Geometry check sheet. Reference: the model listing, model coordinates, mm. A direction names the side the tool comes from. Round coordinates to 2 decimals unless told otherwise and drop trailing zeros. Order: outer loops, then holes, each group sorted by start corner. A loop starts at its lowest first (then second) coordinate and runs counter-clockwise, first axis right, second up. Notation, with made-up numbers: (28.25, 84) - (47.25, 84) arc R23 cw to (47.25, 96) - close; hole circle Ø5 at (-8.5, 74.25). An arc over 180 degrees is marked (long way). Write each question's results on one line, items separated by ' | '.
```python
from build123d import *

# Parameters (mm, degrees)
F0_W     = 38.1
F0_H     = 241.3
F0_W_2   = 57.15
F0_W_3   = 441.96
F1_DEPTH = 12.7
F0_H_2   = 19.05
F2_DEPTH = 12.7


# Not quite as in the source:
# - a feature names something its author has since deleted; it is built from what else it names


with BuildPart() as f1:
    # F0 (on Top) → F1 (new body)
    with BuildSketch(Plane.XY):
        with Locations((-278.13, 0)):
            Rectangle(F0_W, F0_H)
        with Locations((-230.505, 0)):
            Rectangle(F0_W_2, F0_H)
        with Locations((19.05, 0)):
            Rectangle(F0_W_3, F0_H)
        with Locations((268.605, 0)):
            Rectangle(F0_W_2, F0_H)
    extrude(amount=-F1_DEPTH)

    # F0 (on Top) → F2 (join)
    with BuildSketch(Plane.XY):
        with Locations((-230.505, 130.175)):
            Rectangle(F0_W_2, F0_H_2)
        with Locations((-230.505, -130.175)):
            Rectangle(F0_W_2, F0_H_2)
        with Locations((-230.505, 0)):
            Rectangle(F0_W_2, F0_H)
        with Locations((268.605, 0)):
            Rectangle(F0_W_2, F0_H)
        with Locations((268.605, -130.175)):
            Rectangle(F0_W_2, F0_H_2)
        with Locations((268.605, 130.175)):
            Rectangle(F0_W_2, F0_H_2)
    extrude(amount=F2_DEPTH)


solid = f1.part
```
(1) Section check B-B (y = 9). Record the cut outline in (x, z).
Answers follow:
outline: (-297.18, -12.7) - (297.18, -12.7) - (297.18, 12.7) - (240.03, 12.7) - (240.03, 0) - (-201.93, 0) - (-201.93, 12.7) - (-259.08, 12.7) - (-259.08, 0) - (-297.18, 0) - close
(2) Depth check by flat-ended pin: pin 1 Ø6.5 at (y, z) = (-55.5, 6) entering from -X; pin 2 Ø21 at (x, y) = (-232, 132.5) entering from -Z; pin 3 Ø11.5 at (x, y) = (-270.5, 24.5) entering from +Z. Enter the tip coordinate at first touch or a pass-through.
Answers follow:
pin 1: x = -259.08 | pin 2: z = 0 | pin 3: z = 0
(3) Section check A-A (z = 6). Record the cut outline in (x, y).
Answers follow:
outline: (-259.08, -139.7) - (-201.93, -139.7) - (-201.93, 139.7) - (-259.08, 139.7) - close; (240.03, -139.7) - (297.18, -139.7) - (297.18, 139.7) - (240.03, 139.7) - close
(4) Section check C-C (x = -176). Record the cut outline in (y, z), then the cut area to 3 significant figures.
Answers follow:
outline: (-120.65, -12.7) - (120.65, -12.7) - (120.65, 0) - (-120.65, 0) - close | area: 3,060 mm²
(5) Access from +Z, -Z, +X, -X, +Y, -Y to the whole of each face (thin tool, end or side, straight path). Record for faces 1 (the face through (-4, -120.65, -6)), 2 (the face through (297.18, -2, 0)), 3 (the face through (-278, 2, 0)), 4 (the face through (240.03, 2, 6)), 5 (the face through (-297.18, -2, -6)).
Answers follow:
face 1: -Z, +X, -X, -Y | face 2: +Z, -Z, +X, +Y, -Y | face 3: +Z, -X, +Y, -Y | face 4: +Z, +Y, -Y | face 5: +Z, -Z, -X, +Y, -Y
(6) Material ranges on line 1 (X direction, y = 48, z = 4.5); line 2 (Z direction, x = 237, y = 12); line 3 (Y direction, x = 32, z = -9), recorded low to high.
Answers follow:
line 1: -259.08 to -201.93, 240.03 to 297.18 | line 2: -12.7 to 0 | line 3: -120.65 to 120.65
(7) Draft check along X on faces 6 (the face through (4, 120.65, -6)), 7 (the face through (-259.08, 2, 6)), 8 (the face through (16, 2, 0)). Enter one of: released by +X, released by -X, zero draft, split by the parting line, or undercut.
Answers follow:
face 6: zero draft | face 7: released by -X | face 8: undercut
